Print and shaded views of the part. All mm, measured from the part's lowest x, y and z. Round coordinates to 2 decimals unless told otherwise and drop trailing zeros. Order: outer loops, then holes, each group sorted by start corner. A loop starts at its lowest first (then second) coordinate and runs counter-clockwise, first axis right, second up. Notation, with made-up numbers: (-30, 60) -> (-23, 60) arc R28 cw to (-23, 97) -> close; hole circle Ø2 at (-30.5, 89.25). An arc over 180 degrees is marked (long way). Answer as CSV lines item,"result". Start each with the question number.
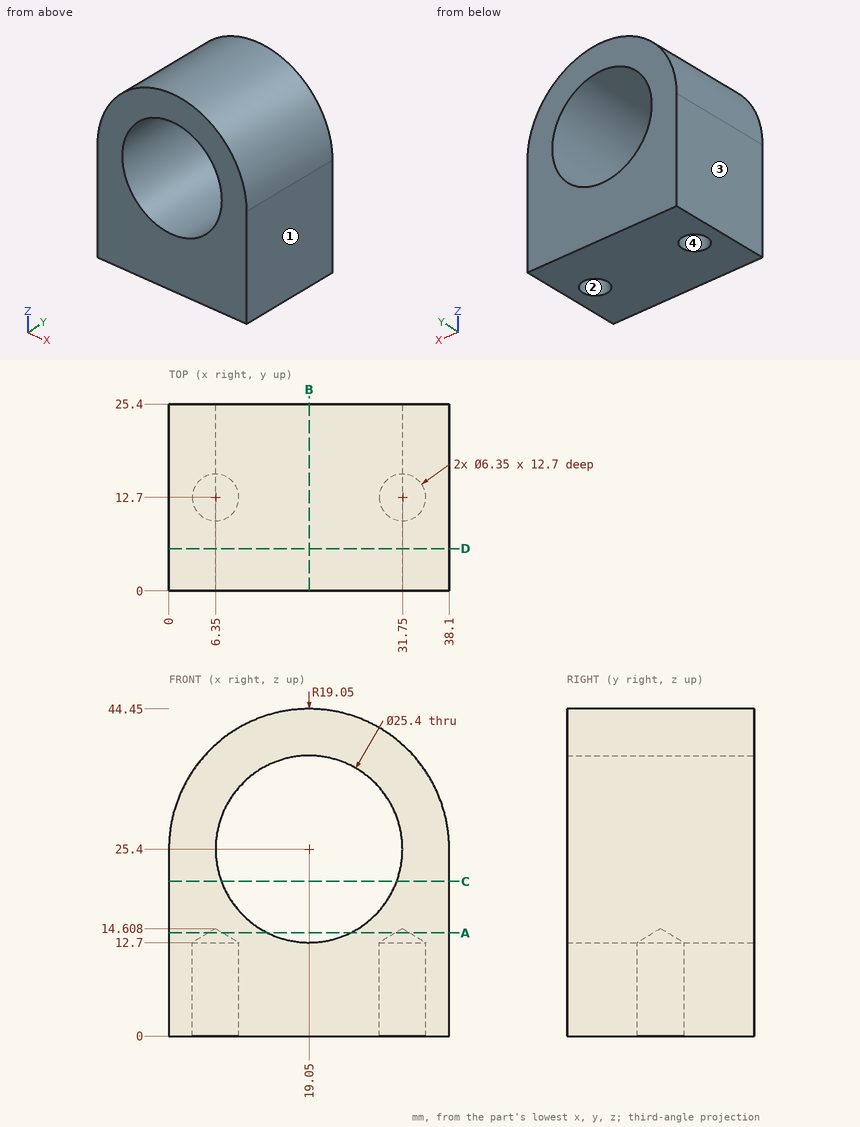
Item 1: Band-saw the part on C-C, the plane z = 21. Give the cut face in (x, y).
Item 2: Band-saw the part on B-B, the plane x = 19.05. Give the cut face in (y, z).
Item 3: Pin check, flat tips, straight feed: pin 1 (6 mm diameter, centred on x = 5, y = 7, fed in from +Z); pin 2 (2 mm diameter, centred on y = 8, z = 30.5, fed in from +X); pin 3 (4 mm diameter, centred on x = 31.75, y = 12.7, fed in from +Z). Stop position of each tip, or through.
Item 4: Probe line 1 (X direction, y = 12.7, z = 8) (1 decimal); line 2 (X direction, y = 15.5, z = 4) (1 decimal); line 3 (Z direction, x = 19.05, y = 12.5). List the from-to ranges inside material, lowest first.
Item 5: Mould opens along X. For the marked faces 1, 2, 3 and 4 say: released by +X, released by -X, zero draft, split by the parting line, or undercut.
Item 6: Band-saw the part on D-D, the plane y = 5.75. Give the cut face in (x, z), and give its area (3 significant figures).
Item 7: Band-saw the part on A-A, the plane z = 14. Give the cut face in (x, y).
Values:
1,outline,"(0, 0) -> (7.14, 0) -> (7.14, 25.4) -> (0, 25.4) -> close; (30.96, 0) -> (38.1, 0) -> (38.1, 25.4) -> (30.96, 25.4) -> close"
2,outline,"(0, 0) -> (25.4, 0) -> (25.4, 12.7) -> (0, 12.7) -> close; (0, 38.1) -> (25.4, 38.1) -> (25.4, 44.45) -> (0, 44.45) -> close"
3,pin 1,"z = 40.92"
3,pin 2,"x = 37.65"
3,pin 3,"z = 41.16"
4,line 1,"0 to 3.2, 9.5 to 28.6, 34.9 to 38.1"
4,line 2,"0 to 4.9, 7.8 to 30.3, 33.2 to 38.1"
4,line 3,"0 to 12.7, 38.1 to 44.45"
5,face 1,"released by +X"
5,face 2,"undercut"
5,face 3,"released by -X"
5,face 4,"undercut"
6,outline,"(0, 0) -> (38.1, 0) -> (38.1, 25.4) arc R19.05 ccw to (0, 25.4) -> close; hole circle Ø25.4 at (19.05, 25.4)"
6,area,"1,030 mm²"
7,outline,"(0, 0) -> (13.45, 0) -> (13.45, 25.4) -> (0, 25.4) -> close; (24.65, 0) -> (38.1, 0) -> (38.1, 25.4) -> (24.65, 25.4) -> close; hole circle Ø2.02 at (6.35, 12.7); hole circle Ø2.02 at (31.75, 12.7)"
